Read the model definition and answer for the solid it produces. Units are mm, in the model's axes. A direction names the side the tool comes from. Coordinates: 2 decimals unless noted, no trailing zeros. Order: outer loops, then holes, each group sorted by start corner. A loop starts at its lowest first (then second) coordinate and runs counter-clockwise, first axis right, second up. Notation, with made-up numbers: (61.5, 59) -> (104.5, 59) arc R25 cw to (104.5, 84) -> close; hole circle Ø9 at (-26.75, 88.25). An arc over 180 degrees is marked (long way). Answer in a Markdown table with one row per item.
from build123d import *

# Parameters (mm, degrees)
FLANGE_BASE1_DEPTH    = 63
ESBO_O6_R             = 19.05
CORTE_EXTRUS_O1_DEPTH = 20
CORTE_EXTRUS_O2_REACH = 71.419
ESBO_O7_R             = 4.5


# Sheet-metal steps are written as plain solids
with BuildPart() as part:
    # Esboço1 → Flange-base1 (new body)
    with BuildSketch(Plane.XY):
        with BuildLine():
            Line((0, 0), (0, 22.2))
            ThreePointArc((0, 22.2), (0.820101013, 24.179898987), (2.8, 25))
            Line((2.8, 25), (12.2, 25))
            ThreePointArc((12.2, 25), (14.179898987, 24.179898987), (15, 22.2))
            Line((15, 22.2), (15, 0))
            Line((15, 0), (13.2, 0))
            Line((13.2, 0), (13.2, 22.2))
            ThreePointArc((13.2, 22.2), (12.907106781, 22.907106781), (12.2, 23.2))
            Line((12.2, 23.2), (2.8, 23.2))
            ThreePointArc((2.8, 23.2), (2.092893219, 22.907106781), (1.8, 22.2))
            Line((1.8, 22.2), (1.8, 0))
            Line((1.8, 0), (0, 0))
        make_face()
    extrude(amount=FLANGE_BASE1_DEPTH)

    # Esboço6 → Corte-extrusão1 (cut)
    with BuildSketch(Plane(origin=(15, 0, 0), x_dir=(0, 0, -1), z_dir=(1, 0, 0))):
        with Locations((-31.5, 0)):
            Circle(ESBO_O6_R)
    extrude(amount=-CORTE_EXTRUS_O1_DEPTH, mode=Mode.SUBTRACT)

    # Esboço7 → Corte-extrusão2 (cut, up to next)
    with BuildSketch(Plane(origin=(0, 25, 0), x_dir=(1, 0, 0), z_dir=(0, 1, 0)), mode=Mode.PRIVATE) as corte_extrus_o2_sk1:
        with Locations(Location((7.5, -54.55, 0), (0, 0, 270))):
            Circle(ESBO_O7_R)
    corte_extrus_o2_tool1 = extrude(corte_extrus_o2_sk1.sketch, amount=-CORTE_EXTRUS_O2_REACH, mode=Mode.PRIVATE) & part.part
    # Esboço7 → Corte-extrusão2 (cut, up to next)
    with BuildSketch(Plane(origin=(0, 25, 0), x_dir=(1, 0, 0), z_dir=(0, 1, 0)), mode=Mode.PRIVATE) as corte_extrus_o2_sk2:
        with Locations(Location((7.5, -8.45, 0), (0, 0, 270))):
            Circle(ESBO_O7_R)
    corte_extrus_o2_tool2 = extrude(corte_extrus_o2_sk2.sketch, amount=-CORTE_EXTRUS_O2_REACH, mode=Mode.PRIVATE) & part.part
    add(corte_extrus_o2_tool1.solids().sort_by_distance((7.5, 25, 54.55))[0], mode=Mode.SUBTRACT)
    add(corte_extrus_o2_tool2.solids().sort_by_distance((7.5, 25, 8.45))[0], mode=Mode.SUBTRACT)


solid = part.part
Q1. The part is cut by section B-B (z = 8.45). Write down the section's boundary in (x, y).
Outcome:
| item | result |
|---|---|
| outline | (0, 0) -> (1.8, 0) -> (1.8, 22.2) arc R1 cw to (2.8, 23.2) -> (3, 23.2) -> (3, 25) -> (2.8, 25) arc R2.8 ccw to (0, 22.2) -> close; (12, 23.2) -> (12.2, 23.2) arc R1 cw to (13.2, 22.2) -> (13.2, 0) -> (15, 0) -> (15, 22.2) arc R2.8 ccw to (12.2, 25) -> (12, 25) -> close |
Q2. For faces 5 (the face through (14.113, 19.045, 31.081)), 6 (the face through (8, 23.2, 31)), determine the directions among +Z, -Z, +X, -X, +Y, -Y from which every point of the face is accessible in a straight line to the end or side of a thin tool.
Outcome:
| item | result |
|---|---|
| face 5 | +X, -X, -Y |
| face 6 | +Z, -Z, -Y |
Q3. For a pull along X with two mould halves and no side action, classify faces 1 (the face through (8.852, 24.113, 58.842)), 2 (the face through (1.8, 21, 31)), 3 (the face through (15, 21, 31)), 4 (the face through (1, 0, 57)) as pulls with the +X half, pulls with the -X half, needs draft (parallel to the pull), parting line crosses it, or undercut.
Outcome:
| item | result |
|---|---|
| face 1 | undercut |
| face 2 | undercut |
| face 3 | pulls with the +X half |
| face 4 | needs draft |
Q4. Consider line 1 (X direction, y = 2.5, z = 52); line 2 (Z direction, x = 6.5, y = 24.25); line 3 (Y direction, x = 4, z = 48). Determine where each line is inside the solid, lowest interval first.
Outcome:
| item | result |
|---|---|
| line 1 | 0 to 1.8, 13.2 to 15 |
| line 2 | 0 to 4.06, 12.84 to 50.16, 58.94 to 63 |
| line 3 | 23.2 to 25 |
Q5. The part is cut by section D-D (z = 29). Write down the section's boundary in (x, y).
Outcome:
| item | result |
|---|---|
| outline | (0, 18.89) -> (1.8, 18.89) -> (1.8, 22.2) arc R1 cw to (2.8, 23.2) -> (12.2, 23.2) arc R1 cw to (13.2, 22.2) -> (13.2, 18.89) -> (15, 18.89) -> (15, 22.2) arc R2.8 ccw to (12.2, 25) -> (2.8, 25) arc R2.8 ccw to (0, 22.2) -> close |
Q6. The part is cut by section A-A (x = 7.5). Write down the section's boundary in (y, z).
Outcome:
| item | result |
|---|---|
| outline | (23.2, 0) -> (25, 0) -> (25, 3.95) -> (23.2, 3.95) -> close; (23.2, 12.95) -> (25, 12.95) -> (25, 50.05) -> (23.2, 50.05) -> close; (23.2, 59.05) -> (25, 59.05) -> (25, 63) -> (23.2, 63) -> close |
Q7. Given pin 1 (3 mm diameter, centred on x = 5.5, z = 25.5, fed in from -Y), flat-ended and moving along its own axis, determine where the tip first touches the part or whether it passes through.
Outcome:
| item | result |
|---|---|
| pin 1 | y = 23.2 |
Q8. The part is cut by section C-C (y = 3.5). Write down the section's boundary in (x, z).
Outcome:
| item | result |
|---|---|
| outline | (0, 0) -> (1.8, 0) -> (1.8, 12.77) -> (0, 12.77) -> close; (0, 50.23) -> (1.8, 50.23) -> (1.8, 63) -> (0, 63) -> close; (13.2, 0) -> (15, 0) -> (15, 12.77) -> (13.2, 12.77) -> close; (13.2, 50.23) -> (15, 50.23) -> (15, 63) -> (13.2, 63) -> close |
